Here's how the part is built. I have some questions about the finished solid (model axes, mm). A direction names the side the tool comes from. Round coordinates to 2 decimals unless told otherwise and drop trailing zeros. Loops run counter-clockwise (first coordinate to the right, second up) from the corner with the lowest first, then second, coordinate; pieces in that order, holes last. Notation, with made-up numbers: M -33,78 L 1,78 A17 cw 1,91 Z; hole C 46,-17 d8. An arc over 180 degrees is marked long. Answer as a JSON object with one key per item and string values.
from build123d import *

# Parameters (mm, degrees)
BASE_FLANGE1_DEPTH  = 83
SKETCH2_W           = 50
SKETCH2_H           = 3.1
SKETCH2_W_2         = 25
BOSS_EXTRUDE1_DEPTH = 3
SKETCH3_W           = 138
SKETCH3_H           = 3.2
SKETCH3_W_2         = 25
BOSS_EXTRUDE2_DEPTH = 3
CUT_EXTRUDE1_REACH  = 337.928
SKETCH4_R           = 5.25
SKETCH4_W           = 21.2
SKETCH4_H           = 30


# Sheet-metal steps are written as plain solids
with BuildPart() as part:
    # Sketch1 → Base-Flange1 (new body)
    with BuildSketch(Plane(origin=(0, 0, 0), x_dir=(1, 0, 0), z_dir=(0, 1, 0))):
        with BuildLine():
            Line((-144, 137), (-126.171572875, 154.828427125))
            ThreePointArc((-126.171572875, 154.828427125), (-124.87387948, 155.69551813), (-123.343145751, 156))
            Line((-123.343145751, 156), (123.343145751, 156))
            ThreePointArc((123.343145751, 156), (124.87387948, 155.69551813), (126.171572875, 154.828427125))
            Line((126.171572875, 154.828427125), (142.828427125, 138.171572875))
            ThreePointArc((142.828427125, 138.171572875), (143.69551813, 136.87387948), (144, 135.343145751))
            Line((144, 135.343145751), (144, -135))
            Line((144, -135), (141, -135))
            Line((141, -135), (141, 135.343145751))
            ThreePointArc((141, 135.343145751), (140.923879533, 135.725829183), (140.707106781, 136.050252532))
            Line((140.707106781, 136.050252532), (124.050252532, 152.707106781))
            ThreePointArc((124.050252532, 152.707106781), (123.725829183, 152.923879533), (123.343145751, 153))
            Line((123.343145751, 153), (-123.343145751, 153))
            ThreePointArc((-123.343145751, 153), (-123.725829183, 152.923879533), (-124.050252532, 152.707106781))
            Line((-124.050252532, 152.707106781), (-141.878679656, 134.878679656))
            Line((-141.878679656, 134.878679656), (-144, 137))
        make_face()
    extrude(amount=BASE_FLANGE1_DEPTH)

    # Sketch2 → Boss-Extrude1 (add)
    with BuildSketch(Plane(origin=(0, 0, -156), x_dir=(-1, 0, 0), z_dir=(0, 0, -1))):
        with Locations((0, -1.55)):
            Rectangle(SKETCH2_W, SKETCH2_H)
        with Locations((-87.5, -1.55)):
            Rectangle(SKETCH2_W_2, SKETCH2_H)
        with Locations((87.5, -1.55)):
            Rectangle(SKETCH2_W_2, SKETCH2_H)
    boss_extrude1 = extrude(amount=-BOSS_EXTRUDE1_DEPTH)

    # Sketch3 → Boss-Extrude2 (add)
    with BuildSketch(Plane(origin=(144, 0, 0), x_dir=(0, 0, -1), z_dir=(1, 0, 0))):
        with Locations((0, -1.6)):
            Rectangle(SKETCH3_W, SKETCH3_H)
        with Locations((106.5, -1.6)):
            Rectangle(SKETCH3_W_2, SKETCH3_H)
        with Locations((-106.5, -1.6)):
            Rectangle(SKETCH3_W_2, SKETCH3_H)
    boss_extrude2 = extrude(amount=-BOSS_EXTRUDE2_DEPTH)

    # Mirror1: Boss-Extrude1, Boss-Extrude2 across plane
    add(boss_extrude1.mirror(Plane.ZX.offset(41.5)))
    add(boss_extrude2.mirror(Plane.ZX.offset(41.5)))

    # Sketch4 → Cut-Extrude1 (cut, up to next)
    with BuildSketch(Plane(origin=(0, 0, -156), x_dir=(-1, 0, 0), z_dir=(0, 0, -1)), mode=Mode.PRIVATE) as cut_extrude1_sk1:
        with Locations((-80, 59.5)):
            Circle(SKETCH4_R)
    cut_extrude1_tool1 = extrude(cut_extrude1_sk1.sketch, amount=-CUT_EXTRUDE1_REACH, mode=Mode.PRIVATE) & part.part
    # Sketch4 → Cut-Extrude1 (cut, up to next)
    with BuildSketch(Plane(origin=(0, 0, -156), x_dir=(-1, 0, 0), z_dir=(0, 0, -1)), mode=Mode.PRIVATE) as cut_extrude1_sk2:
        with Locations((-105, 59.5)):
            Rectangle(SKETCH4_W, SKETCH4_H)
    cut_extrude1_tool2 = extrude(cut_extrude1_sk2.sketch, amount=-CUT_EXTRUDE1_REACH, mode=Mode.PRIVATE) & part.part
    add(cut_extrude1_tool1.solids().sort_by_distance((80, 59.5, -156))[0], mode=Mode.SUBTRACT)
    add(cut_extrude1_tool2.solids().sort_by_distance((105, 59.5, -156))[0], mode=Mode.SUBTRACT)


solid = part.part
Item 1: I'm going to push flat-ended pins straight in: pin 1 Ø2.5 at (x, z) = (103, -154) entering from +Y; pin 2 Ø0.9 at (y, z) = (-2, -154.5) entering from +X; pin 3 Ø4 at (y, z) = (44.5, -50) entering from -X. Where does each tip first touch, or does it pass through?
Resolved:
{"pin 1": "y = 83", "pin 2": "x = 100", "pin 3": "x = 141"}
Item 2: I want a section at C-C, the plane y = 28. Please give me the cut outline in (x, z).
Resolved:
{"outline": "M -144,-137 L -126.17,-154.83 A4 ccw -123.34,-156 L 123.34,-156 A4 ccw 126.17,-154.83 L 142.83,-138.17 A4 ccw 144,-135.34 L 144,135 L 141,135 L 141,-135.34 A1 cw 140.71,-136.05 L 124.05,-152.71 A1 cw 123.34,-153 L -123.34,-153 A1 cw -124.05,-152.71 L -141.88,-134.88 Z"}
Item 3: On a 3-axis mill with a long thin cutter (end or side, diameter ignored), from which of +Z, -Z, +X, -X, +Y, -Y can I reach the whole of each face in a straight line? I mean faces 1 (the face through (2, 41, -153)), 2 (the face through (-125, 83, -152)), 3 (the face through (-125, 0, -152)). Say none if no direction works.
Resolved:
{"face 1": "+Z, +Y, -Y", "face 2": "+Z, -Z, -X, +Y", "face 3": "+Z, -Z, -X, -Y"}
Item 4: I want a section at B-B, the plane x = 107. Please give me the cut outline in (y, z).
Resolved:
{"outline": "M 0,-156 L 44.5,-156 L 44.5,-153 L 0,-153 Z; M 74.5,-156 L 83,-156 L 83,-153 L 74.5,-153 Z"}
Item 5: If we mould it in two halves opening along X, with no side actions, what happens to faces 4 (the face through (134, 41, -147)), 5 (the face through (77.58, 54.84, -154.52)), 6 (the face through (132, 0, -146))? For each: pulls with the +X half, pulls with the -X half, needs draft (parallel to the pull), parting line crosses it, or undercut.
Resolved:
{"face 4": "pulls with the +X half", "face 5": "undercut", "face 6": "needs draft"}
Item 6: I want a section at A-A, the plane y = 59.5. Please give me the cut outline in (x, z).
Resolved:
{"outline": "M -144,-137 L -126.17,-154.83 A4 ccw -123.34,-156 L 74.75,-156 L 74.75,-153 L -123.34,-153 A1 cw -124.05,-152.71 L -141.88,-134.88 Z; M 85.25,-156 L 94.4,-156 L 94.4,-153 L 85.25,-153 Z; M 115.6,-156 L 123.34,-156 A4 ccw 126.17,-154.83 L 142.83,-138.17 A4 ccw 144,-135.34 L 144,135 L 141,135 L 141,-135.34 A1 cw 140.71,-136.05 L 124.05,-152.71 A1 cw 123.34,-153 L 115.6,-153 Z"}
Item 7: I want a section at D-D, the plane z = -89. Please give me the cut outline in (x, y), then the cut area to 3 significant figures.
Resolved:
{"outline": "M 141,0 L 144,0 L 144,83 L 141,83 Z", "area": "249 mm²"}
Item 8: Please list where these lines run through material, in increasing order: probe 1 along Y at (x, z) = (80, -153.75); probe 2 along X at (y, z) = (59, -154); probe 3 along X at (y, z) = (74, -32). Write a range as from..to.
Resolved:
{"probe 1": "-3.1..54.25, 64.75..86.1", "probe 2": "-127..74.77, 85.23..94.4, 115.6..127", "probe 3": "141..144"}
